Build history of the part. All positions in model axes, mm. Round coordinates to 2 decimals unless told otherwise and drop trailing zeros. Write each loop counter-clockwise with the first axis right and the second up, starting at its lowest first coordinate (ties: lowest second). Pieces come first, ordered by that corner, then holes. Notation, with made-up numbers: M 48.5,63.5 L 93.5,63.5 A27 cw 93.5,87.5 Z; hole C 54,3 d6. An arc over 180 degrees is marked long. Use a Markdown table: item, result.
from build123d import *

# Parameters (mm, degrees)
SKETCH1_R           = 1.63195
BOSS_EXTRUDE1_DEPTH = 6.35


with BuildPart() as part:
    # Sketch1 → Boss-Extrude1 (new body)
    with BuildSketch(Plane(origin=(0, 0, 0), x_dir=(1, 0, 0), z_dir=(0, 1, 0))):
        with BuildLine():
            Line((0, -11), (0, -76.2))
            Line((0, -76.2), (76.22, -76.2))
            Line((76.22, -76.2), (76.22, 76.2))
            Line((76.22, 76.2), (0, 76.2))
            Line((0, 76.2), (0, 11))
            ThreePointArc((0, 11), (11, 0), (0, -11))
        make_face()
        with Locations(Location((69.87, 69.85, 0), (0, 0, 270))):
            Circle(SKETCH1_R, mode=Mode.SUBTRACT)
        with Locations(Location((69.87, -69.85, 0), (0, 0, 90))):
            Circle(SKETCH1_R, mode=Mode.SUBTRACT)
        with Locations(Location((50.82, 69.85, 0), (0, 0, 270))):
            Circle(SKETCH1_R, mode=Mode.SUBTRACT)
        with Locations(Location((25.42, 69.85, 0), (0, 0, 270))):
            Circle(SKETCH1_R, mode=Mode.SUBTRACT)
        with Locations(Location((50.82, -69.85, 0), (0, 0, 90))):
            Circle(SKETCH1_R, mode=Mode.SUBTRACT)
        with Locations(Location((25.42, -69.85, 0), (0, 0, 90))):
            Circle(SKETCH1_R, mode=Mode.SUBTRACT)
    extrude(amount=BOSS_EXTRUDE1_DEPTH)


solid = part.part
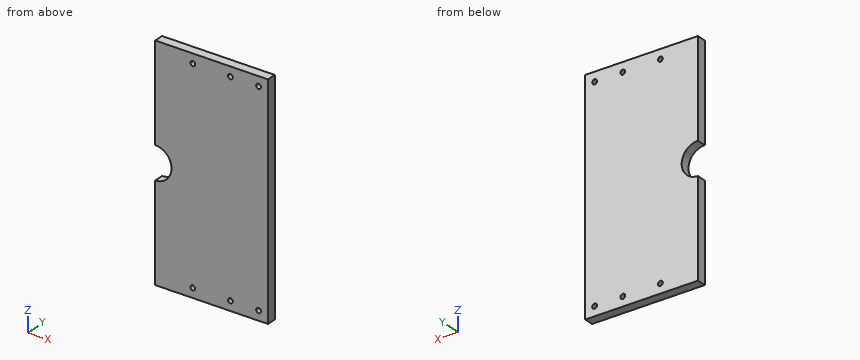
Q1. Drop a flat-ended pin along its axis: P1, Ø5, axis at x = 25.42, z = 69.85, coming from the +Y side. Give the stop position or say it passes through.
Response values:
| item | result |
|---|---|
| P1 | stops at y = 6.35 |
Q2. Cut at A-A on z = -69.85. Give the cut face in (x, y), and give its area (3 significant figures).
Response values:
| item | result |
|---|---|
| outline | M 0,0 L 23.79,0 L 23.79,6.35 L 0,6.35 Z; M 27.05,0 L 49.19,0 L 49.19,6.35 L 27.05,6.35 Z; M 52.45,0 L 68.24,0 L 68.24,6.35 L 52.45,6.35 Z; M 71.5,0 L 76.22,0 L 76.22,6.35 L 71.5,6.35 Z |
| area | 422 mm2 |
Q3. Cut at C-C on x = 69.87. Give the cut face in (y, z).
Response values:
| item | result |
|---|---|
| outline | M 0,-76.2 L 6.35,-76.2 L 6.35,-71.48 L 0,-71.48 Z; M 0,-68.22 L 6.35,-68.22 L 6.35,68.22 L 0,68.22 Z; M 0,71.48 L 6.35,71.48 L 6.35,76.2 L 0,76.2 Z |
Q4. Cut at B-B on y = 3. Give the cut face in (x, z).
Response values:
| item | result |
|---|---|
| outline | M 0,-76.2 L 76.22,-76.2 L 76.22,76.2 L 0,76.2 L 0,11 A11 cw 0,-11 Z; hole C 25.42,-69.85 d3.26; hole C 25.42,69.85 d3.26; hole C 50.82,-69.85 d3.26; hole C 50.82,69.85 d3.26; hole C 69.87,-69.85 d3.26; hole C 69.87,69.85 d3.26 |
Q5. Drill centre lines: L1, parallel to X at y = 4.5, z = -69.85; L2, parallel to Z at x = 8.5, y = 6; L3, parallel to X at y = 2, z = -8.5. Where is each one in solid material? Low to high.
Response values:
| item | result |
|---|---|
| L1 | x = 0 to 23.79, 27.05 to 49.19, 52.45 to 68.24, 71.5 to 76.22 |
| L2 | z = -76.2 to -6.98, 6.98 to 76.2 |
| L3 | x = 6.98 to 76.22 |
